from build123d import *

# Parameters (mm, degrees)
F0_W         = 50.8
F0_H         = 50.8
F1_DEPTH     = 30
F2_W         = 50.8
F2_H         = 50.8
F3_DEPTH     = 30
F5_R         = 10
F4_R         = 14
F8_DEPTH     = 7
F10_DEPTH    = 5.9
F12_DEPTH    = 7
F13_T1_DEPTH = 9.3614920568
F13_T3_DEPTH = 9.3614920568
F14_R        = 1


# Not quite as in the source:
# - a fillet or chamfer that OpenCascade refuses, or shapes differently, is made with other operations: its cross-section is extruded or revolved along the edge and cut away or added


with BuildPart() as f1:
    # F0 (on Top) → F1 (new body)
    with BuildSketch(Plane.XY):
        Rectangle(F0_W, F0_H)
    extrude(amount=F1_DEPTH)

    # F2 (on face) → F3 (cut, through all)
    with BuildSketch(Plane.XY.offset(30)):
        Rectangle(F2_W, F2_H)
        with BuildLine():
            ThreePointArc((-12.8399150562, 1.7135403152), (-11.7164214446, 2.5724711068), (-10.857490653, 1.4489774952))
            ThreePointArc((-10.857490653, 1.4489774952), (-10.9296586704, 0.7260856773), (-10.95375, 0))
            Line((-10.95375, 0), (10.95375, 0))
            ThreePointArc((10.95375, 0), (10.9296586704, 0.7260856773), (10.857490653, 1.4489774952))
            ThreePointArc((10.857490653, 1.4489774952), (11.7164214446, 2.5724711068), (12.8399150562, 1.7135403152))
            Line((12.8399150562, 1.7135403152), (15.08125, -15.08125))
            Line((15.08125, -15.08125), (15.08125, -18.25625))
            Line((15.08125, -18.25625), (-15.08125, -18.25625))
            Line((-15.08125, -18.25625), (-15.08125, -15.08125))
            Line((-15.08125, -15.08125), (-12.8399150562, 1.7135403152))
        make_face(mode=Mode.SUBTRACT)
        with BuildLine():
            Line((10.95375, 0), (-10.95375, 0))
            ThreePointArc((-10.95375, 0), (0, -10.95375), (10.95375, 0))
        make_face()
    extrude(amount=-F3_DEPTH, mode=Mode.SUBTRACT)

    # F5 (on Front) → F6 section 0
    with BuildSketch(Plane.XZ):
        with Locations((0, 15)):
            Circle(F5_R)
    # F4 (on face) → F6 section 1
    with BuildSketch(Plane.XZ.offset(18.25625)):
        with Locations((0, 15)):
            Circle(F4_R)
    loft(mode=Mode.SUBTRACT)

    # F7 (on face) → F8 (join)
    with BuildSketch(Plane.XY.offset(30)):
        with BuildLine():
            ThreePointArc((-10.857490653, 1.4489774952), (-10.9287333274, 1.9732487889), (-11.2575085067, 2.3877880386))
            ThreePointArc((-11.2575085067, 2.3877880386), (-12.2406927383, 2.5012284324), (-12.8399150562, 1.7135403152))
            Line((-12.8399150562, 1.7135403152), (-15.08125, -15.08125))
            Line((-15.08125, -15.08125), (-15.08125, -18.25625))
            Line((-15.08125, -18.25625), (15.08125, -18.25625))
            Line((15.08125, -18.25625), (15.08125, -15.08125))
            Line((15.08125, -15.08125), (12.8399150562, 1.7135403152))
            ThreePointArc((12.8399150562, 1.7135403152), (12.2406927383, 2.5012284324), (11.2575085067, 2.3877880386))
            ThreePointArc((11.2575085067, 2.3877880386), (10.9287333274, 1.9732487889), (10.857490653, 1.4489774952))
            ThreePointArc((10.8574906531, 1.4489774952), (0, -10.95375), (-10.857490653, 1.4489774952))
        make_face()
        with BuildLine():
            ThreePointArc((8, 0), (0, -8), (-8, 0))
            Line((-8, 0), (-11.2575085067, 2.3877880386))
            ThreePointArc((-11.2575085067, 2.3877880386), (-10.9287333274, 1.9732487889), (-10.857490653, 1.4489774952))
            ThreePointArc((-10.857490653, 1.4489774952), (0, -10.95375), (10.8574906531, 1.4489774952))
            ThreePointArc((10.857490653, 1.4489774952), (10.9287333274, 1.9732487889), (11.2575085067, 2.3877880386))
            Line((11.2575085067, 2.3877880386), (8, 0))
        make_face()
    extrude(amount=F8_DEPTH)

    # F9 (on face) → F10 (join)
    with BuildSketch(Plane.XY.offset(37)):
        with BuildLine():
            ThreePointArc((8, 0), (0, -8), (-8, 0))
            Line((-8, 0), (-13.0685941712, 0))
            Line((-13.0685941712, 0), (-15.08125, -15.08125))
            Line((-15.08125, -15.08125), (-15.08125, -18.25625))
            Line((-15.08125, -18.25625), (15.08125, -18.25625))
            Line((15.08125, -18.25625), (15.08125, -15.08125))
            Line((15.08125, -15.08125), (13.0685941712, 0))
            Line((13.0685941712, 0), (8, 0))
        make_face()
        with BuildLine():
            ThreePointArc((6, 0), (0, -6), (-6, 0))
            Line((-6, 0), (-8, 0))
            ThreePointArc((-8, 0), (0, -8), (8, 0))
            Line((8, 0), (6, 0))
        make_face()
    extrude(amount=F10_DEPTH)

    # F11 (on face) → F12 (join)
    with BuildSketch(Plane.XY.offset(42.9)):
        with BuildLine():
            Line((11.2575085067, 2.3877880386), (8, 0))
            Line((8, 0), (13.0685941712, 0))
            Line((13.0685941712, 0), (12.8399150562, 1.7135403152))
            ThreePointArc((12.8399150562, 1.7135403152), (12.2406927383, 2.5012284324), (11.2575085067, 2.3877880386))
        make_face()
        with BuildLine():
            Line((-13.0685941712, 0), (-8, 0))
            Line((-8, 0), (-11.2575085067, 2.3877880386))
            ThreePointArc((-11.2575085067, 2.3877880386), (-12.2406927383, 2.5012284324), (-12.8399150562, 1.7135403152))
            Line((-12.8399150562, 1.7135403152), (-13.0685941712, 0))
        make_face()
        with BuildLine():
            ThreePointArc((8, 0), (0, -8), (-8, 0))
            Line((-8, 0), (-13.0685941712, 0))
            Line((-13.0685941712, 0), (-15.08125, -15.08125))
            Line((-15.08125, -15.08125), (-15.08125, -18.25625))
            Line((-15.08125, -18.25625), (15.08125, -18.25625))
            Line((15.08125, -18.25625), (15.08125, -15.08125))
            Line((15.08125, -15.08125), (13.0685941712, 0))
            Line((13.0685941712, 0), (8, 0))
        make_face()
    extrude(amount=F12_DEPTH)

    # F13: fillet of radius 2 on 4 edges, made by hand

    # F13_s2 → F13_t1 (cut)
    with BuildSketch(Plane.XY.offset(42.9)):
        with BuildLine():
            ThreePointArc((-7.9553868421, -0.8436943713), (-8.2105441596, -0.0574614627), (-8.7618448568, 0.5584403027))
            Line((-8.7618448568, 0.5584403027), (-8, 0))
            ThreePointArc((-8, 0), (-7.9888389249, -0.4224365414), (-7.9553868421, -0.8436943713))
        make_face()
        with BuildLine():
            ThreePointArc((7.9553868421, -0.8436943713), (8.2105441596, -0.0574614627), (8.7618448568, 0.5584403027))
            Line((8.7618448568, 0.5584403027), (8, 0))
            ThreePointArc((8, 0), (7.9888389249, -0.4224365414), (7.9553868421, -0.8436943713))
        make_face()
    extrude(amount=F13_T1_DEPTH, mode=Mode.SUBTRACT)

    # F13_s4 → F13_t3 (cut)
    with BuildSketch(Plane.XY.offset(27.6385079432)):
        with BuildLine():
            ThreePointArc((-7.9553868421, -0.8436943713), (-8.2105441596, -0.0574614627), (-8.7618448568, 0.5584403027))
            Line((-8.7618448568, 0.5584403027), (-8, 0))
            ThreePointArc((-8, 0), (-7.9888389249, -0.4224365414), (-7.9553868421, -0.8436943713))
        make_face()
        with BuildLine():
            ThreePointArc((7.9553868421, -0.8436943713), (8.2105441596, -0.0574614627), (8.7618448568, 0.5584403027))
            Line((8.7618448568, 0.5584403027), (8, 0))
            ThreePointArc((8, 0), (7.9888389249, -0.4224365414), (7.9553868421, -0.8436943713))
        make_face()
    extrude(amount=F13_T3_DEPTH, mode=Mode.SUBTRACT)

    # F14
    f14_edges = [f1.edges().sort_by_distance(p)[0] for p in [
        (-6, 0, 39.95),
        (6, 0, 39.95),
    ]]
    fillet(f14_edges, radius=F14_R)


solid = f1.part
Read the model definition and answer for the solid it produces. Units are mm, in the model's axes. A direction names the side the tool comes from. Give positions to 0.01 mm unless a question says otherwise; leave off trailing zeros. Loops run counter-clockwise (first coordinate to the right, second up) from the corner with the lowest first, then second, coordinate; pieces in that order, holes last. Notation, with made-up numbers: (23, -30) -> (78, -30) arc R17 cw to (78, -14) -> close; hole circle Ø4 at (13, -30). An arc over 180 degrees is marked (long way). Use a Markdown table: item, result.
Q1. Section D-D, the plane y = -4.5 is taken. Determine the outline of the cut face in (x, z).
Solved:
| item | result |
|---|---|
| outline | (-13.67, 0) -> (-9.99, 0) -> (-9.99, 10.42) arc R10.99 cw to (-9.99, 19.58) -> (-9.99, 30) -> (-6.61, 30) -> (-6.61, 37) -> (-3.97, 37) -> (-3.97, 42.9) -> (-6.61, 42.9) -> (-6.61, 49.9) -> (-13.67, 49.9) -> close; (3.97, 37) -> (6.61, 37) -> (6.61, 30) -> (9.99, 30) -> (9.99, 19.58) arc R10.99 cw to (9.99, 10.42) -> (9.99, 0) -> (13.67, 0) -> (13.67, 49.9) -> (6.61, 49.9) -> (6.61, 42.9) -> (3.97, 42.9) -> close |
Q2. Section B-B, the plane y = -2 is taken. Determine the outline of the cut face in (x, z), then the cut area to 3 significant figures.
Solved:
| item | result |
|---|---|
| outline | (-13.34, 0) -> (-10.77, 0) -> (-10.77, 30) -> (-7.75, 30) -> (-7.75, 37) -> (-5.66, 37) -> (-5.66, 42.9) -> (-7.75, 42.9) -> (-7.75, 49.9) -> (-13.34, 49.9) -> close; (5.66, 37) -> (7.75, 37) -> (7.75, 30) -> (10.77, 30) -> (10.77, 0) -> (13.34, 0) -> (13.34, 49.9) -> (7.75, 49.9) -> (7.75, 42.9) -> (5.66, 42.9) -> close |
| area | 401 mm^2 |
Q3. Each of these flat-tipped pins is pushed along its axis until it touches: pin 1 (2 mm diameter, centred on x = -11.5, y = 1.5, fed in from -Z); pin 2 (12 mm diameter, centred on x = 5.5, z = 18, fed in from +Y); pin 3 (2.5 mm diameter, centred on x = -2, y = -4.5, fed in from +Z); pin 4 (3 mm diameter, centred on x = 2.5, y = -0.5, fed in from -Z). Where does it stop, or does it pass through?
Solved:
| item | result |
|---|---|
| pin 1 | stops at z = 0 |
| pin 2 | stops at y = 2.52 |
| pin 3 | stops at z = 42.9 |
| pin 4 | passes through |
Q4. A tool of negligible diameter and unlimited length cuts with its end or side. For faces 4 (the face through (10.03, 1.49, 46.35)), 5 (the face through (8.205, -0.068, 46.351)), 6 (the face through (11, 1, 42.9)), 7 (the face through (0, -10, 49.9)), 8 (the face through (8.205, -0.068, 33.451)), from which of +Z, -Z, +X, -X, +Y, -Y can it reach the whole face along a straight path? Write none if from no direction.
Solved:
| item | result |
|---|---|
| face 4 | +Z, -Z, +Y |
| face 5 | +Z, +Y |
| face 6 | +X, -X, +Y |
| face 7 | +Z, +X, -X, +Y, -Y |
| face 8 | -Z, +Y |
Q5. Determine the mould class of faces 1 (the face through (15.081, -17, 25)), 2 (the face through (6.266, -0.251, 39.991)), 3 (the face through (0, -12, 0)) for opening direction X: pulls with the +X half, pulls with the -X half, needs draft (parallel to the pull), parting line crosses it, or undercut.
Solved:
| item | result |
|---|---|
| face 1 | pulls with the +X half |
| face 2 | undercut |
| face 3 | needs draft |
Q6. Section C-C, the plane y = -9.75 is taken. Determine the outline of the cut face in (x, z).
Solved:
| item | result |
|---|---|
| outline | (-14.37, 0) -> (-4.99, 0) -> (-4.99, 3.94) arc R12.14 cw to (-4.99, 26.06) -> (-4.99, 30) -> (4.99, 30) -> (4.99, 26.06) arc R12.14 cw to (4.99, 3.94) -> (4.99, 0) -> (14.37, 0) -> (14.37, 49.9) -> (-14.37, 49.9) -> close |
Q7. Section A-A, the plane x = 0 is taken. Determine the outline of the cut face in (y, z).
Solved:
| item | result |
|---|---|
| outline | (-18.26, 0) -> (-10.95, 0) -> (-10.95, 2.6) -> (-18.26, 1) -> close; (-18.26, 29) -> (-10.95, 27.4) -> (-10.95, 30) -> (-8, 30) -> (-8, 37) -> (-6, 37) -> (-6, 42.9) -> (-8, 42.9) -> (-8, 49.9) -> (-18.26, 49.9) -> close |
Q8. Find the intervals of material crossed by line 1 along Z through (x, y) = (11, 1); line 2 along X through (y, z) = (-15, 12.5); line 3 along X through (y, z) = (-3.5, 9.5), in increasing order.
Solved:
| item | result |
|---|---|
| line 1 | z = 0 to 37, 42.9 to 49.9 |
| line 2 | x = -15.07 to -13.05, 13.05 to 15.07 |
| line 3 | x = -13.54 to -10.38, 10.38 to 13.54 |
